Can you work these out from the model? Positions are in its coordinate system, mm. Face numbers are marked on the shaded views. Give positions to 0.01 mm unless a question says otherwise; leave off trailing zeros. Order: outer loops, then holes, each group sorted by start corner. A loop starts at its lowest first (then second) coordinate and runs counter-clockwise, first axis right, second up.
Item 1: I want a section at C-C, the plane z = 0. Write out the boundary of the cut face in (x, y).
Item 2: I want a section at A-A, the plane z = 25.4. Write out the boundary of the cut face in (x, y).
Item 3: I want a section at B-B, the plane y = -2.5. Count the separate pieces of the cut face and the enclosed holes in it, then the cut area to 3 significant figures.
Item 4: If we mould it in two halves opening along Z, with no side actions, what happens to the marked faces 1 and 2? For each: +Z half, -Z half, draft (parallel to the pull), parting line (faces both ways), or undercut.
Item 5: I want a section at D-D, the plane x = 0. Write out the boundary of the cut face in (y, z), then the cut area to 3 significant figures.
Item 6: If I drill on line 1 along Z through (x, y) = (0, -2.1); line 2 along X through (y, z) = (2.6, 0); line 3 along X through (y, z) = (-1.8, -25.4), over which ranges is the centre line in solid material (lowest first)?
Item 7: I'm going to push flat-ended pins straight in: pin 1 Ø3 at (y, z) = (-2.5, -11.5) entering from -X; pin 2 Ø4 at (y, z) = (-1, -24) entering from +X; pin 3 Ø1.9 at (x, y) = (8.5, -2) entering from +Z. Where does each tip first touch, or does it pass through?
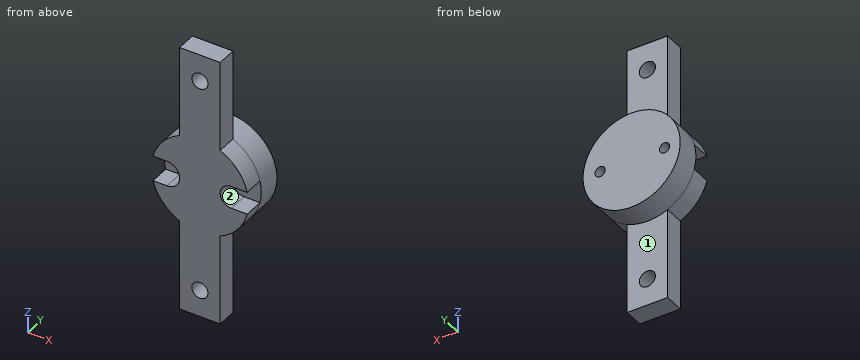
```python
from build123d import *

# Parameters (mm, degrees)
SKETCH1_R             = 11.43
SKETCH1_R_2           = 1.2
BOSS_EXTRUDE1_DEPTH   = 5.7785
BOSS_EXTRUDE2_DEPTH   = 4.671568
F_6_CLEARANCE_HOLE1_D = 3.7973


with BuildPart() as part:
    # Sketch1 → Boss-Extrude1 (new body)
    with BuildSketch(Plane(origin=(0, 0, 0), x_dir=(1, 0, 0), z_dir=(0, 1, 0))):
        Circle(SKETCH1_R)
        with Locations((-7.75, 0)):
            Circle(SKETCH1_R_2, mode=Mode.SUBTRACT)
        with Locations((7.4, 0)):
            Circle(SKETCH1_R_2, mode=Mode.SUBTRACT)
    extrude(amount=BOSS_EXTRUDE1_DEPTH)

    # Sketch2 → Boss-Extrude2 (add)
    with BuildSketch(Plane.XZ):
        with BuildLine():
            Line((-7.75, -2.9875), (-11.032667119, -2.9875))
            ThreePointArc((-11.032667119, -2.9875), (-8.721989857, -7.387272361), (-4.7625, -10.390548289))
            Line((-4.7625, -10.390548289), (-4.7625, -31.75))
            Line((-4.7625, -31.75), (4.7625, -31.75))
            Line((4.7625, -31.75), (4.7625, -10.390548289))
            ThreePointArc((4.7625, -10.390548289), (8.837593826, -7.248574713), (11.121532887, -2.6375))
            Line((11.121532887, -2.6375), (7.4, -2.6375))
            ThreePointArc((7.4, -2.6375), (4.7625, 0), (7.4, 2.6375))
            Line((7.4, 2.6375), (11.121532887, 2.6375))
            ThreePointArc((11.121532887, 2.6375), (8.837593826, 7.248574713), (4.7625, 10.390548289))
            Line((4.7625, 10.390548289), (4.7625, 31.75))
            Line((4.7625, 31.75), (-4.7625, 31.75))
            Line((-4.7625, 31.75), (-4.7625, 10.390548289))
            ThreePointArc((-4.7625, 10.390548289), (-8.721989857, 7.387272361), (-11.032667119, 2.9875))
            Line((-11.032667119, 2.9875), (-7.75, 2.9875))
            ThreePointArc((-7.75, 2.9875), (-4.7625, 0), (-7.75, -2.9875))
        make_face()
    extrude(amount=BOSS_EXTRUDE2_DEPTH)

    # #6 Clearance Hole1 (through all)
    with Locations(Plane(origin=(0, -4.671568, 0), x_dir=(-1, 0, 0), z_dir=(0, -1, 0))):
        with Locations((0, 25.4), (0, -25.4)):
            Hole(F_6_CLEARANCE_HOLE1_D / 2)


solid = part.part
```
Results list:
1. outline: (-11.43, 0) - (-8.95, 0) - (-8.95, 5.78) - (-11.43, 5.78) - close; (-6.55, 0) - (-4.76, 0) - (-4.76, -4.67) - (4.76, -4.67) - (4.76, 0) - (6.2, 0) - (6.2, 5.78) - (-6.55, 5.78) - close; (8.6, 0) - (11.43, 0) - (11.43, 5.78) - (8.6, 5.78) - close
2. outline: (-4.76, -4.67) - (-1.9, -4.67) - (-1.9, 0) - (-4.76, 0) - close; (1.9, -4.67) - (4.76, -4.67) - (4.76, 0) - (1.9, 0) - close
3. separate pieces: 1
3. enclosed holes: 2
3. area: 714 mm2
4. face 1: draft
4. face 2: undercut
5. outline: (-4.67, -31.75) - (0, -31.75) - (0, -27.3) - (-4.67, -27.3) - close; (-4.67, -23.5) - (0, -23.5) - (0, -11.43) - (5.78, -11.43) - (5.78, 11.43) - (0, 11.43) - (0, 23.5) - (-4.67, 23.5) - close; (-4.67, 27.3) - (0, 27.3) - (0, 31.75) - (-4.67, 31.75) - close
5. area: 393 mm2
6. line 1: z = -31.75 to -27.3, -23.5 to 23.5, 27.3 to 31.75
6. line 2: x = -11.43 to -8.95, -6.55 to 6.2, 8.6 to 11.43
6. line 3: x = -4.76 to -1.9, 1.9 to 4.76
7. pin 1: stops at x = -5.54
7. pin 2: stops at x = 4.76
7. pin 3: stops at z = 8.58
